from build123d import *

# Parameters (mm, degrees)
SKETCH_1_W          = 40
SKETCH_1_H          = 9
EXTRUDE_1_DEPTH     = 5
SKETCH_2_R          = 2.75
CUT_EXTRUDE_1_DEPTH = 10
SKETCH_3_R          = 2.5
CUT_EXTRUDE_2_DEPTH = 10


with BuildPart() as part:
    # 草图1 → 凸台-拉伸1 (new body)
    with BuildSketch(Plane.XY):
        with Locations((0, 4.5)):
            Rectangle(SKETCH_1_W, SKETCH_1_H)
    extrude(amount=EXTRUDE_1_DEPTH)

    # 草图2 → 切除-拉伸1 (cut)
    with BuildSketch(Plane.XY.offset(5)):
        with Locations((15, 4.5)):
            Circle(SKETCH_2_R)
        with Locations((-15, 4.5)):
            Circle(SKETCH_2_R)
    extrude(amount=-CUT_EXTRUDE_1_DEPTH, mode=Mode.SUBTRACT)

    # 草图3 → 切除-拉伸2 (cut)
    with BuildSketch(Plane(origin=(0, 9, 0), x_dir=(1, 0, 0), z_dir=(0, 1, 0))):
        with Locations((0, -6)):
            Circle(SKETCH_3_R)
    extrude(amount=-CUT_EXTRUDE_2_DEPTH, mode=Mode.SUBTRACT)


solid = part.part
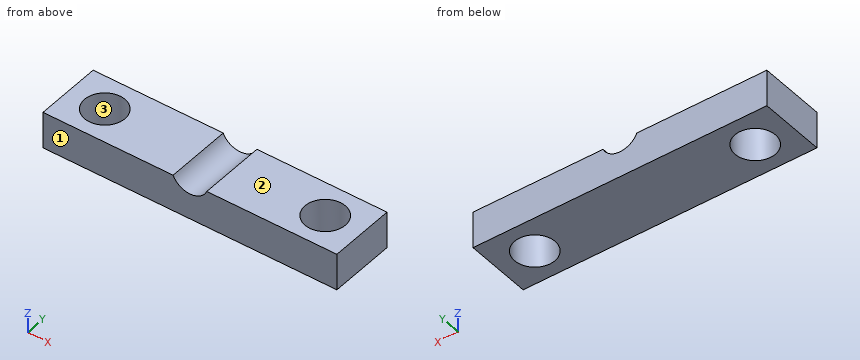
Input: part model. Units: mm. Frame: model coordinates. Face numbers are marked on the shaded views. Coordinates: 2 decimals unless noted, no trailing zeros. Loops run counter-clockwise (first coordinate to the right, second up) from the corner with the lowest first, then second, coordinate; pieces in that order, holes last.
(1) Section B-B on y = 4.5. Return the cut outline in (x, z).
(2) Section C-C on x = -17. Return the cut outline in (y, z).
(3) Section D-D on y = 1.25. Return the cut outline in (x, z), then the cut area to 3 significant figures.
(4) First-contact query: pin 1 Ø3.5 at (x, y) = (-15, 4.5) entering from -Z; pin 2 Ø1.5 at (x, y) = (-16, 2) entering from -Z. Flat tips, straight axial feed; report the tip coordinate or a pass-through.
(5) Pull-direction query (Y, two-part tool) for the marked faces 1, 2 and 3; classes: released by +Y, released by -Y, zero draft, split by the parting line, or undercut.
(6) Section A-A on z = 0.6. Return the cut outline in (x, y), then the cut area to 3 significant figures.
(7) Material intervals for probe 1 along X at (y, z) = (5.5, 1.5); probe 2 along Y at (x, z) = (15, 1.95); probe 3 along X at (y, z) = (3, 3.85), sorted ascending.
Data:
1. outline: (-20, 0) - (-17.75, 0) - (-17.75, 5) - (-20, 5) - close; (-12.25, 0) - (12.25, 0) - (12.25, 5) - (2.29, 5) arc R2.5 cw to (-2.29, 5) - (-12.25, 5) - close; (17.75, 0) - (20, 0) - (20, 5) - (17.75, 5) - close
2. outline: (0, 0) - (2.61, 0) - (2.61, 5) - (0, 5) - close; (6.39, 0) - (9, 0) - (9, 5) - (6.39, 5) - close
3. outline: (-20, 0) - (20, 0) - (20, 5) - (2.29, 5) arc R2.5 cw to (-2.29, 5) - (-20, 5) - close
3. area: 195 mm2
4. pin 1: passes through
4. pin 2: stops at z = 0
5. face 1: released by -Y
5. face 2: zero draft
5. face 3: undercut
6. outline: (-20, 0) - (20, 0) - (20, 9) - (-20, 9) - close; hole circle Ø5.5 at (-15, 4.5); hole circle Ø5.5 at (15, 4.5)
6. area: 312 mm2
7. probe 1: x = -20 to -17.56, -12.44 to 12.44, 17.56 to 20
7. probe 2: y = 0 to 1.75, 7.25 to 9
7. probe 3: x = -20 to -17.3, -12.7 to -1.28, 1.28 to 12.7, 17.3 to 20
